Part model, mm, in its own coordinate system. Round coordinates to 2 decimals unless told otherwise and drop trailing zeros. Write each loop counter-clockwise with the first axis right and the second up, starting at its lowest first coordinate (ties: lowest second). Pieces come first, ordered by that corner, then holes. Notation, with made-up numbers: M 21,89 L 59,89 A19 cw 59,116 Z; hole C -39,48.5 d11. An arc over 180 degrees is marked long. One line per question, with ' | ' between items. Start each with the question number.
1) Saw through at A-A (z = 0). List the corners of the cut face in (x, y).
2) Drop flat-ended pins along their axis: pin 1 Ø2.5 at (x, z) = (0, 0) entering from -Y; pin 2 Ø1 at (x, y) = (-8.5, 0) entering from -Z. Give the stop position or say it passes through.
3) Saw through at B-B (y = 0.7). List the corners of the cut face in (x, z).
4) Saw through at C-C (x = -39.5). List the corners of the cut face in (y, z), plus the area to 3 significant figures.
5) Saw through at D-D (z = -2.25). List the corners of the cut face in (x, y), plus the area to 3 significant figures.
6) Mould opens along Z. For faces 1 (the face through (2.75, 0.01, -0.06)), 2 (the face through (-25, -1, 0)), 3 (the face through (0.45, 0.01, 1.43)) say: pulls with the +Z half, pulls with the -Z half, needs draft (parallel to the pull), parting line crosses it, or undercut.
7) Wall check: probe 1 along X at (y, z) = (0, 0); probe 2 along X at (y, z) = (-0.25, -1); probe 3 along Z at (x, y) = (-2.5, -0.1). Give the ranges that are in metal, low to high. Write a range as [from, to].
```python
from build123d import *

# Parameters (mm, degrees)
SKETCH1_R           = 1.5
BOSS_EXTRUDE1_DEPTH = 20
SKETCH2_R           = 1.5
BOSS_EXTRUDE2_DEPTH = 1
SKETCH3_R           = 1.5
CUT_EXTRUDE1_DEPTH  = 68.268120235


with BuildPart() as part:
    # Sketch1 → Boss-Extrude1 (new, symmetric)
    with BuildSketch(Plane(origin=(0, 0, 0), x_dir=(1, 0, 0), z_dir=(0, 1, 0))):
        with Locations(Location((0, 0, 0), (0, 0, 270))):
            Circle(SKETCH1_R)
    extrude(amount=BOSS_EXTRUDE1_DEPTH, both=True)

    # Sketch2 → Boss-Extrude2 (add, symmetric)
    with BuildSketch(Plane(origin=(0, 0, 0), x_dir=(1, 0, 0), z_dir=(0, 1, 0))):
        with BuildLine():
            Line((-50.985294118, 2.999963956), (0.013480392, 2.74996696))
            ThreePointArc((0.013480392, 2.74996696), (2.75, 0), (0.013480392, -2.74996696))
            Line((0.013480392, -2.74996696), (-50.985294118, -2.999963956))
            ThreePointArc((-50.985294118, -2.999963956), (-54, 0), (-50.985294118, 2.999963956))
        make_face()
        with Locations(Location((-51, 0, 0), (0, 0, 270))):
            Circle(SKETCH2_R, mode=Mode.SUBTRACT)
    extrude(amount=BOSS_EXTRUDE2_DEPTH, both=True)

    # Sketch3 → Cut-Extrude1 (cut, through all)
    with BuildSketch(Plane(origin=(0, 20, 0), x_dir=(1, 0, 0), z_dir=(0, 1, 0))):
        with Locations(Location((0, 0, 0), (0, 0, 270))):
            Circle(SKETCH3_R)
    extrude(amount=-CUT_EXTRUDE1_DEPTH, mode=Mode.SUBTRACT)


solid = part.part
```
Answer key:
1) outline: M -54,-1 L -52.5,-1 L -52.5,1 L -54,1 Z; M -49.5,-1 L -1.5,-1 L -1.5,1 L -49.5,1 Z; M 1.5,-1 L 2.75,-1 L 2.75,1 L 1.5,1 Z
2) pin 1: passes through | pin 2: stops at z = -2.79
3) outline: M -50.99,-3 L 0.01,-2.75 A2.75 ccw 0.01,2.75 L -50.99,3 A3 ccw long Z; hole C -51,0 d3; hole C 0,0 d3
4) outline: M -1,-2.94 L 1,-2.94 L 1,2.94 L -1,2.94 Z | area: 11.8 mm2
5) outline: M -52.98,-1 L 1.58,-1 L 1.58,1 L -52.98,1 Z | area: 109 mm2
6) face 1: parting line crosses it | face 2: needs draft | face 3: undercut
7) probe 1: x = [-54, -52.5], [-49.5, -1.5], [1.5, 2.75] | probe 2: x = [-53.83, -52.12], [-49.88, -1.12], [1.12, 2.56] | probe 3: z = [-2.76, 2.76]
